```python
from build123d import *

# Parameters (mm, degrees)
SKETCH2_W           = 50.8
SKETCH2_H           = 25.4
SKETCH2_W_2         = 44.45
SKETCH2_H_2         = 19.05
BOSS_EXTRUDE1_DEPTH = 622.3
CUT_EXTRUDE1_REACH  = 625.336


with BuildPart() as part:
    # Sketch2 → Boss-Extrude1 (new body)
    with BuildSketch(Plane.XY):
        Rectangle(SKETCH2_W, SKETCH2_H)
        Rectangle(SKETCH2_W_2, SKETCH2_H_2, mode=Mode.SUBTRACT)
    extrude(amount=BOSS_EXTRUDE1_DEPTH)

    # Cut-Extrude1: up to this face of the body (flat: up to its plane)
    cut_extrude1_end = Plane(part.part.faces().sort_by_distance((0, -12.7, 311.15))[0])
    # Sketch3 → Cut-Extrude1 (cut, up to the picked face)
    with BuildSketch(Plane(origin=(0, 12.7, 0), x_dir=(1, 0, 0), z_dir=(0, 1, 0)), mode=Mode.PRIVATE) as cut_extrude1_sk1:
        Polygon((-25.4, -622.3), (25.4, -596.416107166), (25.4, -622.3), align=None)
    cut_extrude1_tool1 = split(extrude(cut_extrude1_sk1.sketch, amount=-CUT_EXTRUDE1_REACH, mode=Mode.PRIVATE), bisect_by=cut_extrude1_end, keep=Keep.BOTH, mode=Mode.PRIVATE)
    add(cut_extrude1_tool1.solids().sort_by(Axis((8.466667, 12.7, 613.672036), (0, -1, 0)))[0], mode=Mode.SUBTRACT)


solid = part.part
```
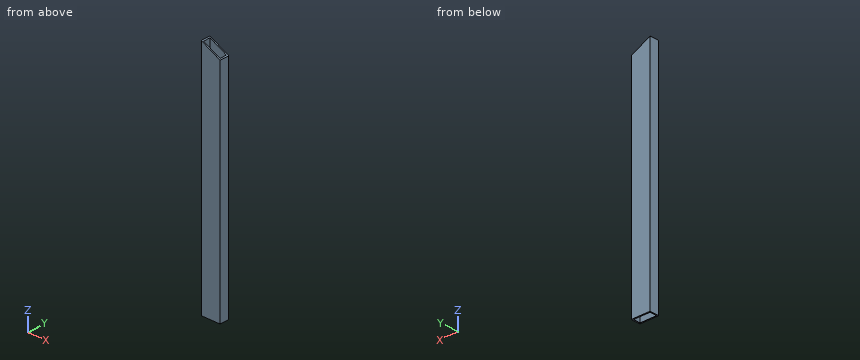
Design review of the part built by this model. Coordinates are the model's own, in mm. Round coordinates to 2 decimals unless told otherwise and drop trailing zeros. Write each loop counter-clockwise with the first axis right and the second up, starting at its lowest first coordinate (ties: lowest second). Pieces come first, ordered by that corner, then holes.
Item 1: We need section A-A on z = 499. Write out the cut boundary in (x, y) (3 decimals), and give its area (3 significant figures).
Item 2: Clearance check with flat-ended pins moving along their axes: pin 1 Ø8 at (x, y) = (6, -8) entering from +Z; pin 2 Ø10 at (x, y) = (7.5, 0) entering from -Z; pin 3 Ø1.5 at (x, y) = (-19.5, 9.5) entering from +Z. State where each tip first meets the part, or that it passes through.
Item 3: We need section C-C on x = -14. Write out the cut boundary in (y, z) (3 decimals).
Item 4: We need section B-B on y = 3. Write out the cut boundary in (x, z) (3 decimals).
Item 5: For probe 1 along Y at (x, z) = (-13, 306) (3 decimals); probe 2 along X at (y, z) = (4, 203.5) (3 decimals), list the stretches that pass through material, from the lowest coordinate up.
Returned:
1. outline: (-25.4, -12.7) - (25.4, -12.7) - (25.4, 12.7) - (-25.4, 12.7) - close; hole (-22.225, -9.525) - (22.225, -9.525) - (22.225, 9.525) - (-22.225, 9.525) - close
1. area: 444 mm2
2. pin 1: stops at z = 608.19
2. pin 2: passes through
2. pin 3: stops at z = 619.68
3. outline: (-12.7, 0) - (-9.525, 0) - (-9.525, 616.491) - (-12.7, 616.491) - close; (9.525, 0) - (12.7, 0) - (12.7, 616.491) - (9.525, 616.491) - close
4. outline: (-25.4, 0) - (-22.225, 0) - (-22.225, 620.682) - (-25.4, 622.3) - close; (22.225, 0) - (25.4, 0) - (25.4, 596.416) - (22.225, 598.034) - close
5. probe 1: y = -12.7 to -9.525, 9.525 to 12.7
5. probe 2: x = -25.4 to -22.225, 22.225 to 25.4
